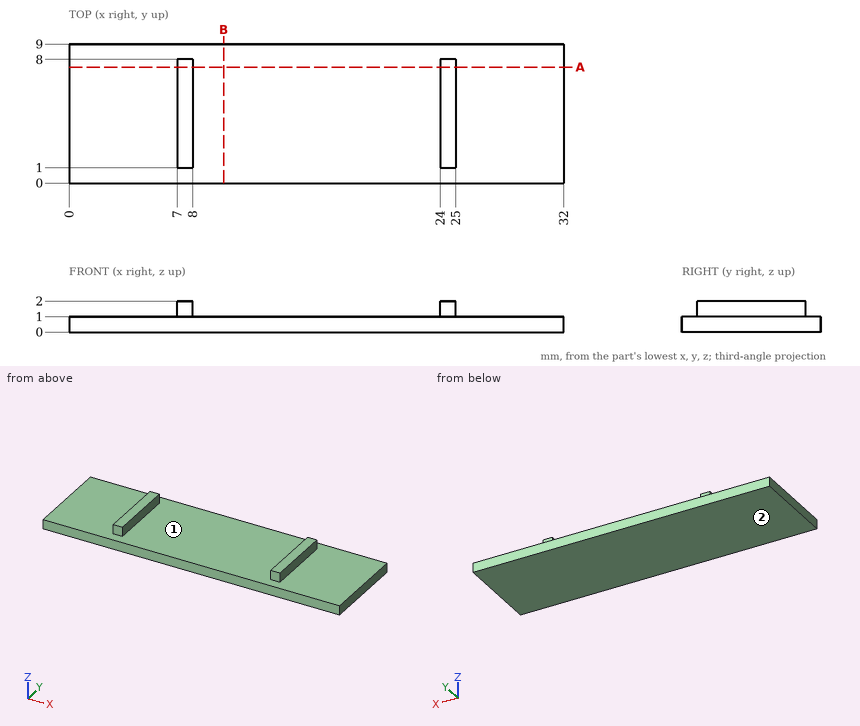
Check sheet for the drawn part. Datum: minimum x, y, z corner. Units: mm. Coordinates: 2 decimals unless noted, no trailing zeros. Write each loop counter-clockwise with the first axis right and the second up, starting at its lowest first coordinate (ties: lowest second). Pieces come first, ordered by that corner, then holes. Notation, with made-up numbers: (8, 23.5) - (29, 23.5) arc R15 ccw to (29, 29.5) - close; hole circle Ø7 at (-4, -28.75). An arc over 180 degrees is marked (long way). Answer as a JSON object with one key per item and string values.
(1) Gauge pin test, flat ends, axial feed: pin 1 Ø0.8 at (x, z) = (7.5, 1.5) entering from +Y; pin 2 Ø0.5 at (y, z) = (4.5, 1.5) entering from -X; pin 3 Ø1.1 at (x, z) = (24.5, 1.5) entering from -Y; pin 4 Ø0.8 at (y, z) = (3, 1.5) entering from +X. Record the tip position at first contact, or that the pin passes through.
Report:
{"pin 1": "y = 8", "pin 2": "x = 7", "pin 3": "y = 0", "pin 4": "x = 25"}
(2) Thickness scan on line 1 along X through (y, z) = (4.5, 1.5); line 2 along Z through (x, y) = (5, 7). Record the ranges inside material, lowest first.
Report:
{"line 1": "7 to 8, 24 to 25", "line 2": "0 to 1"}
(3) Cross-section at B-B on x = 10. Record the cut outline in (y, z), plus the area to 3 significant figures.
Report:
{"outline": "(0, 0) - (9, 0) - (9, 1) - (0, 1) - close", "area": "9.00 mm^2"}
(4) Mould release check, pull along X, two halves, no side actions. Record for the marked faces 1 and 2: pulls with the +X half, pulls with the -X half, needs draft (parallel to the pull), parting line crosses it, or undercut.
Report:
{"face 1": "undercut", "face 2": "needs draft"}
(5) Cross-section at A-A on y = 7.5. Record the cut outline in (x, z).
Report:
{"outline": "(0, 0) - (32, 0) - (32, 1) - (25, 1) - (25, 2) - (24, 2) - (24, 1) - (8, 1) - (8, 2) - (7, 2) - (7, 1) - (0, 1) - close"}
